Could you check a few things on this drawing? It's one solid part, dimensions in mm from its lowest x, y, z. A direction names the side the tool comes from. Coordinates: 2 decimals unless noted, no trailing zeros. Order: outer loops, then holes, each group sorted by start corner. A loop starts at its lowest first (then second) coordinate and runs counter-clockwise, first axis right, second up. Notation, with made-up numbers: (-15.5, 77.5) -> (31.5, 77.5) arc R21 ccw to (31.5, 88.5) -> close; hole circle Ø6 at (70, 89.5). An arc over 180 degrees is marked (long way). Answer as CSV lines item,"result".
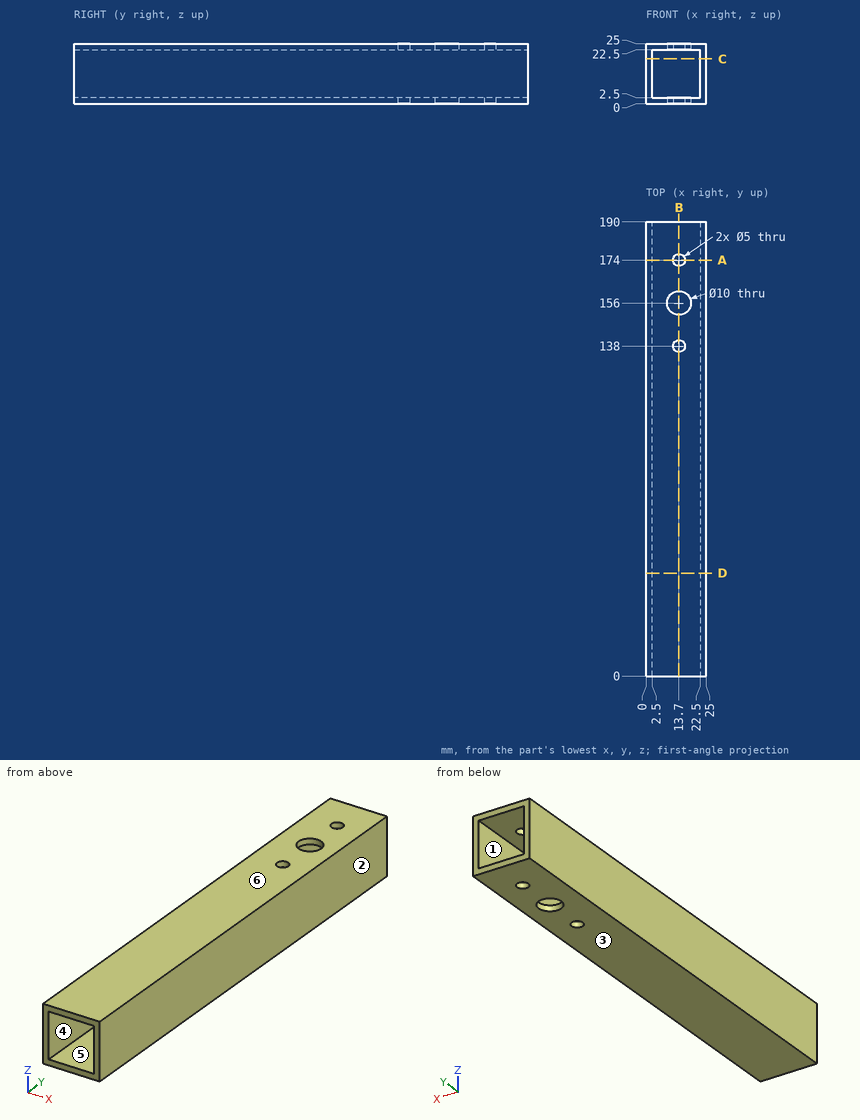
Q1. Which directions (+Z, -Z, +X, -X, +Y, -Y) give clear straight access to the entire face, cutting with the end or side of a thin tool? Please do the marked faces 5 and 6.
Solution:
face 5,"+Y, -Y"
face 6,"+Z, +X, -X, +Y, -Y"
Q2. We'd pull the mould along X, two halves only. Please class the marked faces 1, 2, 3 and 4: pulls with the +X half, pulls with the -X half, needs draft (parallel to the pull), parting line crosses it, or undercut.
Solution:
face 1,"undercut"
face 2,"pulls with the +X half"
face 3,"needs draft"
face 4,"undercut"
Q3. For P1, Ø3, axis at x = 13.7, y = 138, coming from the +Z side, with a flat end and sliding along its axis, tell me the tip position at first contact or that it passes through.
Solution:
P1,"through"
Q4. Imagine slicing it at A-A (y = 174). List the corners of the cut face in (x, z) for me.
Solution:
outline,"(0, 0) -> (11.2, 0) -> (11.2, 2.5) -> (2.5, 2.5) -> (2.5, 22.5) -> (11.2, 22.5) -> (11.2, 25) -> (0, 25) -> close; (16.2, 0) -> (25, 0) -> (25, 25) -> (16.2, 25) -> (16.2, 22.5) -> (22.5, 22.5) -> (22.5, 2.5) -> (16.2, 2.5) -> close"
Q5. Imagine slicing it at B-B (x = 13.7). Give the number of separate pieces and of enclosed holes in the cut face, and give its area (3 significant figures).
Solution:
separate pieces,"8"
enclosed holes,"0"
area,"850 mm2"
Q6. Imagine slicing it at C-C (z = 18.75). List the corners of the cut face in (x, y) for me.
Solution:
outline,"(0, 0) -> (2.5, 0) -> (2.5, 190) -> (0, 190) -> close; (22.5, 0) -> (25, 0) -> (25, 190) -> (22.5, 190) -> close"
Q7. Imagine slicing it at D-D (y = 43). List the corners of the cut face in (x, z) for me, and give its area (3 significant figures).
Solution:
outline,"(0, 0) -> (25, 0) -> (25, 25) -> (0, 25) -> close; hole (2.5, 2.5) -> (22.5, 2.5) -> (22.5, 22.5) -> (2.5, 22.5) -> close"
area,"225 mm2"
Q8. If I drill on line 1 (Y direction, x = 13.7, z = 0.7); line 2 (X direction, y = 148.5, z = 19.25), over which ranges is the centre line in solid material (lowest first)?
Solution:
line 1,"0 to 135.5, 140.5 to 151, 161 to 171.5, 176.5 to 190"
line 2,"0 to 2.5, 22.5 to 25"
